from build123d import *

# Parameters (mm, degrees)
BOSS_EXTRUDE1_DEPTH = 127
FILLET1_R           = 31.75


with BuildPart() as part:
    # Sketch1 → Boss-Extrude1 (new body)
    with BuildSketch(Plane(origin=(0, 0, 0), x_dir=(1, 0, 0), z_dir=(0, 1, 0))):
        Polygon((88.9, 88.9), (88.9, 241.3), (0, 241.3), (0, 0), (241.3, 0), (241.3, 88.9), align=None)
    extrude(amount=BOSS_EXTRUDE1_DEPTH)

    # Fillet1
    fillet1_edges = [part.edges().sort_by_distance(p)[0] for p in [
        (0, 127, -120.65),
        (120.65, 127, 0),
        (120.65, 0, 0),
        (0, 0, -120.65),
    ]]
    fillet(fillet1_edges, radius=FILLET1_R)


solid = part.part
Model file for the job. Use its own axes, mm. A direction names the side the tool comes from. Coordinates: 2 decimals unless noted, no trailing zeros. Write each loop counter-clockwise with the first axis right and the second up, starting at its lowest first coordinate (ties: lowest second). Pieces come first, ordered by that corner, then holes. Notation, with made-up numbers: (1, -33) - (12, -33) arc R21 cw to (12, -11) - close; hole circle Ø7 at (76, 58.25). An arc over 180 degrees is marked (long way). Write each question's results on one line, items separated by ' | '. Start each with the question number.
1) Cut at A-A (x = 146). Write the cut outline in (y, z).
2) 3-axis set-ups, long thin cutter, end or side, ignore diameter. For faces 1 (the face through (122.3, 117.5, -9.1)), 2 (the face through (88.9, 63, -164)): which of +Z, -Z, +X, -X, +Y, -Y reach the whole face in a straight line?
3) Probe line 1 along X through (y, z) = (95.5, -155); line 2 along Z through (x, y) = (115, 45); line 3 along Z through (x, y) = (21, 97). List the from-to ranges inside material, lowest first. Write a range as from..to.
4) Cut at B-B (y = 54.5). Write the cut outline in (x, z), then the cut area to 3 significant figures.
5) Flat gauge pins, fed straight in: P1, Ø4, axis at x = 145, y = 35, coming from the -Z side; P2, Ø1.5, axis at y = 80, z = -181.5, coming from the +X side. Where does each tip first touch, or does it go through?
Returned:
1) outline: (0, -88.9) - (127, -88.9) - (127, -31.75) arc R31.75 ccw to (95.25, 0) - (31.75, 0) arc R31.75 ccw to (0, -31.75) - close
2) face 1: +Z, +X, -X, +Y | face 2: -Z, +X, +Y, -Y
3) line 1: 0..88.9 | line 2: -88.9..0 | line 3: -241.3..-0.05
4) outline: (0, -241.3) - (88.9, -241.3) - (88.9, -88.9) - (241.3, -88.9) - (241.3, 0) - (0, 0) - close | area: 35,000 mm^2
5) P1: z = -88.9 | P2: x = 88.9
